Autodesk Inventor part; units mm, degrees
ref_plane "YZ Plane" through (0, 0, 0) normal (1, 0, 0) x (0, 1, 0)
ref_plane "XZ Plane" through (0, 0, 0) normal (0, 1, 0) x (-1, 0, 0)
ref_plane "XY Plane" through (0, 0, 0) normal (0, 0, 1) x (1, 0, 0)
sketch "スケッチ1" plane through (0, 0, 0) normal (0, 0, 1) x (1, 0, 0)
  circle A0 centre (0, 0) radius 13
  line L0 (-2.6, 12.7373) -> (-31.4, 6.8586)
  line L1 (-2.6, -12.7373) -> (-31.4, -6.8586)
  arc A1 (-31.4, 6.8586) -> (-31.4, -6.8586) centre (-30, 0) ccw
  line L2 (-47, 0) -> (23, 0)
  circle A2 centre (-5.6569, 5.6569) radius 1.6
  circle A3 centre (6.7175, 6.7175) radius 1.6
  circle A4 centre (5.6569, -5.6569) radius 1.6
  circle A5 centre (-6.7175, -6.7175) radius 1.6
  circle A6 centre (0, 0) radius 2
  dimension "d0" = 30
  dimension "d1" = 26
  dimension "d2" = 7
  dimension "d5" = 4
extrude "押し出し1" add sketch "スケッチ1" along normal blind 2.5 contours L2 A6 A0 | A0 L2 A6 | A0 L2 A1 L0 | L1 A1 L2 A0
sketch "スケッチ2" plane through (0, 0, 0) normal (0, 0, -1) x (-1, 0, 0)
  circle A0 centre (30, 0) radius 3
  circle A1 centre (30, 0) radius 1.5
  circle A2 centre (30, 0) radius 3.6
  line L0 (47, 0) -> (-23, 0)
  arc A3 (31.4, -6.8586) -> (31.4, 6.8586) centre (30, 0) ccw
  circle A4 centre (1.1112, 11) radius 0.8
  circle A5 centre (1.1112, -11) radius 0.8
  circle A6 centre (1.1112, 11) radius 2 construction
  circle A7 centre (1.1112, -11) radius 2 construction
  line L1 (2.6, 12.7373) -> (31.4, 6.8586)
  circle A8 centre (5.6569, 5.6569) radius 1.6
  circle A9 centre (5.6569, 5.6569) radius 1.6
  circle A10 centre (6.7175, -6.7175) radius 1.6
  circle A11 centre (5.6569, 5.6569) radius 3 construction
  circle A12 centre (6.7175, -6.7175) radius 3 construction
  point P0 (0, 0)
  dimension "d6" = 6
  dimension "d7" = 3
  dimension "d8" = 7.2
  dimension "d13" = 1.6
  dimension "d15" = 4
  dimension "d16" = 6
  dimension "d18" = 22
extrude "押し出し2" cut sketch "スケッチ2" against normal blind 0.6 contours L0 A1 A0 | L0 A2 A0 | A0 L0 A2 | A0 L0 A1 | L0 A1 | A1 L0
extrude "押し出し3" cut sketch "スケッチ2" against normal up to surface (2.5 mm away) contours L0 A1 A0 | A0 L0 A1 | L0 A1 | A1 L0 | A4 | A5
thread "ねじ1"
thread "ねじ2"
properties part number "Dribler_main"
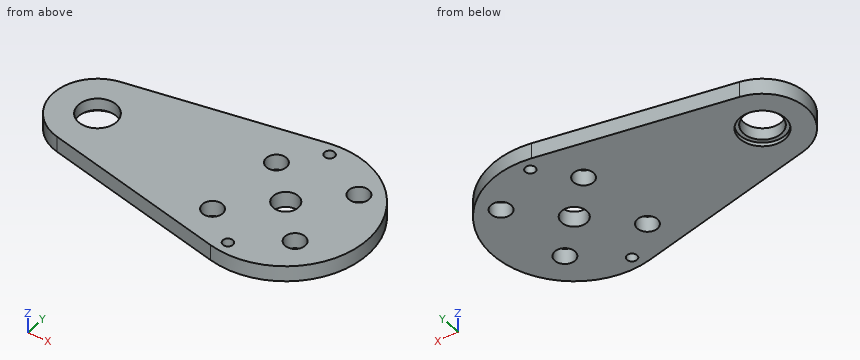
Work out the finished part from the listing and answer in its coordinate system (mm). Round coordinates to 2 decimals unless told otherwise and drop trailing zeros. Write each loop counter-clockwise with the first axis right and the second up, starting at its lowest first coordinate (ties: lowest second). Pieces come first, ordered by that corner, then holes. Notation, with made-up numbers: (-31.5, 34.25) -> (-8.5, 34.25) arc R31 cw to (-8.5, 70.25) -> close; hole circle Ø9 at (78.25, 72.5). An arc over 180 degrees is marked (long way). Write each question's results on one line, items separated by ' | '.
1) The part is cut by section C-C (x = -30). Write down the section's boundary in (y, z).
Findings:
outline: (-7.14, 0) -> (-3.6, 0) -> (-3.6, 0.6) -> (-3, 0.6) -> (-3, 2.5) -> (-7.14, 2.5) -> close; (3, 0.6) -> (3.6, 0.6) -> (3.6, 0) -> (7.14, 0) -> (7.14, 2.5) -> (3, 2.5) -> close
2) The part is cut by section D-D (z = 1.1). State how many separate pieces and enclosed holes the cut face has, and give its area (3 significant figures).
Findings:
separate pieces: 1 | enclosed holes: 8 | area: 877 mm²
3) The part is cut by section B-B (y = -11). Write down the section's boundary in (x, z).
Findings:
outline: (-11.11, 0) -> (-1.91, 0) -> (-1.91, 2.5) -> (-11.11, 2.5) -> close; (-0.31, 0) -> (6.93, 0) -> (6.93, 2.5) -> (-0.31, 2.5) -> close
4) Consider line 1 along Y through (x, z) = (-6, 0.85); line 2 along X through (y, z) = (-1.5, 1.9); line 3 along X through (y, z) = (6.25, 1.9). Determine where each line is inside the solid, lowest interval first. Write a range as [from, to].
Findings:
line 1: y = [-12.04, -8.15], [-5.29, 4.09], [7.22, 12.04] | line 2: x = [-36.84, -32.6], [-27.4, -1.32], [1.32, 12.91] | line 3: x = [-33.15, -7.14], [-4.17, 5.19], [8.25, 11.4]
5) A flat-ended cylindrical pin translates along its axis: pin 1 (3 mm diameter, centred on x = 0, y = 0, fed in from +Z). Find the tip coordinate at first contact, or state that the pin passes through.
Findings:
pin 1: passes through
6) The part is cut by section A-A (y = 0). Write down the section's boundary in (x, z), and give its area (3 significant figures).
Findings:
outline: (-37, 0) -> (-33.6, 0) -> (-33.6, 0.6) -> (-33, 0.6) -> (-33, 2.5) -> (-37, 2.5) -> close; (-27, 0.6) -> (-26.4, 0.6) -> (-26.4, 0) -> (-2, 0) -> (-2, 2.5) -> (-27, 2.5) -> close; (2, 0) -> (13, 0) -> (13, 2.5) -> (2, 2.5) -> close | area: 99.3 mm²
